from build123d import *

# Parameters (mm, degrees)
BOSS_EXTRUDE1_DEPTH = 1.59
SKETCH2_W           = 1.59
SKETCH2_H           = 45
BOSS_EXTRUDE2_DEPTH = 32
SKETCH3_R           = 2.5
SKETCH3_R_2         = 1.75
CUT_EXTRUDE1_DEPTH  = 110.476024773
SKETCH4_R           = 2.5
SKETCH4_R_2         = 1.75
CUT_EXTRUDE2_DEPTH  = 123.822180814


with BuildPart() as part:
    # Sketch1 → Boss-Extrude1 (new body)
    with BuildSketch(Plane.XY):
        with BuildLine():
            Line((0, 14), (-100, 14))
            Line((-100, 14), (-100, -14))
            Line((-100, -14), (0, -14))
            ThreePointArc((0, -14), (14, 0), (0, 14))
        make_face()
    extrude(amount=BOSS_EXTRUDE1_DEPTH)

    # Sketch2 → Boss-Extrude2 (add)
    with BuildSketch(Plane.XY.offset(1.59)):
        with Locations((-99.205, -8.5)):
            Rectangle(SKETCH2_W, SKETCH2_H)
    extrude(amount=BOSS_EXTRUDE2_DEPTH)

    # Sketch3 → Cut-Extrude1 (cut, through all)
    with BuildSketch(Plane.XY.offset(1.59)):
        Circle(SKETCH3_R)
        with Locations((8.5, 0)):
            Circle(SKETCH3_R_2)
        with Locations((-21.25, 0)):
            Circle(SKETCH3_R_2)
        with Locations((-71.82, 0)):
            Circle(SKETCH3_R_2)
    extrude(amount=-CUT_EXTRUDE1_DEPTH, mode=Mode.SUBTRACT)

    # Sketch4 → Cut-Extrude2 (cut, through all)
    with BuildSketch(Plane.ZY.offset(100)):
        with Locations((16.975, 0)):
            Circle(SKETCH4_R)
        with Locations((16.975, 8.5)):
            Circle(SKETCH4_R_2)
        with Locations((16.975, -21.25)):
            Circle(SKETCH4_R_2)
    extrude(amount=-CUT_EXTRUDE2_DEPTH, mode=Mode.SUBTRACT)


solid = part.part
The model under review builds one solid part; all positions refer to its coordinate system, in mm. A direction names the side the tool comes from. Coordinates: 2 decimals unless noted, no trailing zeros. Loops run counter-clockwise (first coordinate to the right, second up) from the corner with the lowest first, then second, coordinate; pieces in that order, holes last.
(1) Consider section B-B, the plane x = -71.82. Give the boundary of the cut face in (y, z).
Determined:
outline: (-14, 0) - (-1.75, 0) - (-1.75, 1.59) - (-14, 1.59) - close; (1.75, 0) - (14, 0) - (14, 1.59) - (1.75, 1.59) - close
(2) Consider section C-C, the plane y = 0. Give the boundary of the cut face in (x, z) (3 decimals).
Determined:
outline: (-100, 0) - (-73.57, 0) - (-73.57, 1.59) - (-98.41, 1.59) - (-98.41, 14.475) - (-100, 14.475) - close; (-100, 19.475) - (-98.41, 19.475) - (-98.41, 33.59) - (-100, 33.59) - close; (-70.07, 0) - (-23, 0) - (-23, 1.59) - (-70.07, 1.59) - close; (-19.5, 0) - (-2.5, 0) - (-2.5, 1.59) - (-19.5, 1.59) - close; (2.5, 0) - (6.75, 0) - (6.75, 1.59) - (2.5, 1.59) - close; (10.25, 0) - (14, 0) - (14, 1.59) - (10.25, 1.59) - close
(3) Consider section A-A, the plane y = -21.25. Give the boundary of the cut face in (x, z) (3 decimals).
Determined:
outline: (-100, 1.59) - (-98.41, 1.59) - (-98.41, 15.225) - (-100, 15.225) - close; (-100, 18.725) - (-98.41, 18.725) - (-98.41, 33.59) - (-100, 33.59) - close
(4) Wall thickness on L1, parallel to X at y = 0, z = 27.5; L2, parallel to Z at x = -39.5, y = -6: over which ranges is each line inside the solid? List them lowest first.
Determined:
L1: x = -100 to -98.41
L2: z = 0 to 1.59
(5) Insertion check: P1, Ø4, axis at x = 1.5, y = 5.5, coming from the +Z side; P2, Ø3, axis at x = -71.82, y = 0, coming from the +Z side; P3, Ø16, axis at y = -0.5, z = 24, coming from the +X side; P4, Ø0.8, axis at x = -99, y = -22, coming from the -Z side. Each pin has a flat end and moves straight along its axis. Give the tip position at first contact, or say it passes through.
Determined:
P1: stops at z = 1.59
P2: passes through
P3: stops at x = -98.41
P4: stops at z = 1.59
(6) Draft analysis for pull direction Y (two halves, no side actions). For faces 3 (the flat face through (-50, 14, 1)), 4 (the flat face through (-100, -9, 17)), 5 (the cylindrical face through (-0.54, -2.44, 0.81)), state which applies: +Y half, -Y half, draft (parallel to the pull), parting line (faces both ways), or undercut.
Determined:
face 3: +Y half
face 4: draft
face 5: undercut
(7) Tool access review of faces 1 (the flat face through (-43, 0, 1.59)), 2 (the cylindrical face through (14, 0, 1)): name each direction out of +Z, -Z, +X, -X, +Y, -Y from which nothing blocks a thin tool from reaching the whole face with its end or side.
Determined:
face 1: +Z, +X, +Y, -Y
face 2: +Z, -Z, +X
(8) Consider section D-D, the plane z = 17. Give the boundary of the cut face in (x, y).
Determined:
outline: (-100, -31) - (-98.41, -31) - (-98.41, -23) - (-100, -23) - close; (-100, -19.5) - (-98.41, -19.5) - (-98.41, -2.5) - (-100, -2.5) - close; (-100, 2.5) - (-98.41, 2.5) - (-98.41, 6.75) - (-100, 6.75) - close; (-100, 10.25) - (-98.41, 10.25) - (-98.41, 14) - (-100, 14) - close
